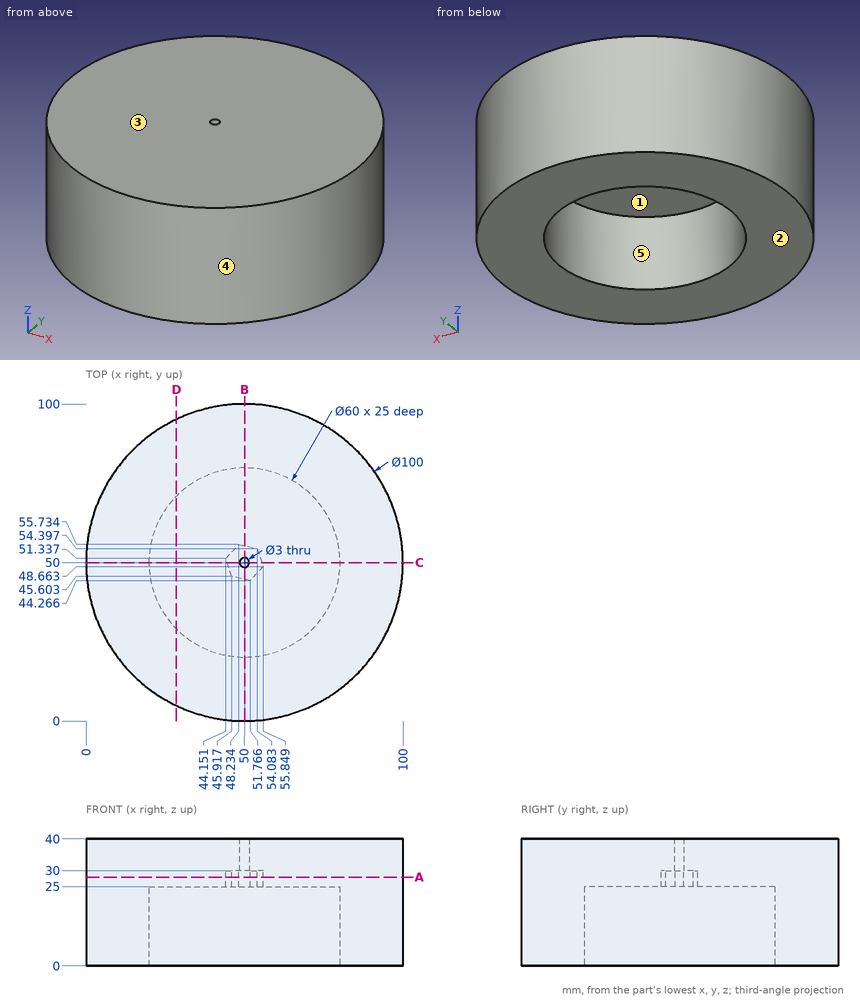
The figure shows three views and two pictorial views of one solid part (mm, origin at its lowest corner). Answer the questions. A direction names the side the tool comes from. Give positions to 0.01 mm unless a question says otherwise; leave off trailing zeros. Write each loop counter-clockwise with the first axis right and the second up, starting at its lowest first coordinate (ties: lowest second). Pieces come first, ordered by that corner, then holes.
Q1. The part is cut by section D-D on x = 28.5. Give the vertices of the cut face in (y, z), and give its area (4 significant figures).
Answer:
outline: (4.86, 0) - (29.08, 0) - (29.08, 25) - (70.92, 25) - (70.92, 0) - (95.14, 0) - (95.14, 40) - (4.86, 40) - close
area: 2,565 mm2
Q2. For a pull along Y with two mould halves and no side action, classify the marked faces 3, 4 and 5 as released by +Y, released by -Y, zero draft, split by the parting line, or undercut.
Answer:
face 3: zero draft
face 4: split by the parting line
face 5: undercut
Q3. The part is cut by section B-B on x = 50. Give the vertices of the cut face in (y, z).
Answer:
outline: (0, 0) - (20, 0) - (20, 25) - (44.67, 25) - (44.67, 30) - (48.5, 30) - (48.5, 40) - (0, 40) - close; (51.5, 30) - (55.33, 30) - (55.33, 25) - (80, 25) - (80, 0) - (100, 0) - (100, 40) - (51.5, 40) - close
Q4. Straight lines are drawn through the part: L1, parallel to Y at x = 50, z = 11; L2, parallel to X at y = 49, z = 6; L3, parallel to Y at x = 50, z = 34. For each, find the intervals that lie inside material, in ascending order.
Answer:
L1: y = 0 to 20, 80 to 100
L2: x = 0.01 to 20.02, 79.98 to 99.99
L3: y = 0 to 48.5, 51.5 to 100
Q5. A tool of negligible diameter and unlimited length cuts with its end or side. For the marked faces 1 and 2, from which of +Z, -Z, +X, -X, +Y, -Y can it reach the whole face along a straight path? Write none if from no direction.
Answer:
face 1: -Z
face 2: -Z, +X, -X, +Y, -Y
Q6. Given pin 1 (4 mm diameter, centred on y = 59, z = 23.5, fed in from +X); pin 2 (5 mm diameter, centred on x = 50, y = 50, fed in from -Z); pin 3 (4 mm diameter, centred on y = 24.5, z = 22.5, fed in from -X), each flat-ended and moving along its own axis, determine where each tip first touches the part or whether it passes through.
Answer:
pin 1: stops at x = 99.51
pin 2: stops at z = 30
pin 3: stops at x = 5.87
Q7. The part is cut by section A-A on z = 28. Give the vertices of the cut face in (x, y) (1 decimal).
Answer:
outline: circle Ø100 at (50, 50); hole (44.2, 51.3) - (45.9, 45.6) - (51.8, 44.3) - (55.8, 48.7) - (54.1, 54.4) - (48.2, 55.7) - close
Q8. The part is cut by section C-C on y = 50. Give the vertices of the cut face in (x, z).
Answer:
outline: (0, 0) - (20, 0) - (20, 25) - (44.56, 25) - (44.56, 30) - (48.5, 30) - (48.5, 40) - (0, 40) - close; (51.5, 30) - (55.44, 30) - (55.44, 25) - (80, 25) - (80, 0) - (100, 0) - (100, 40) - (51.5, 40) - close
